Read the model definition and answer for the solid it produces. Units are mm, in the model's axes. Face numbers are marked on the shaded views. A direction names the side the tool comes from. Coordinates: 2 decimals unless noted, no trailing zeros. Order: outer loops, then holes, each group sorted by start corner. A loop starts at its lowest first (then second) coordinate and runs counter-clockwise, first axis right, second up. Notation, with made-up numbers: (39.25, 53) -> (68.25, 53) arc R22 ccw to (68.25, 64) -> close; hole circle Ø2 at (68.25, 15.25). An arc over 180 degrees is marked (long way). Use CSV: the item, a comma, the result in double quotes.
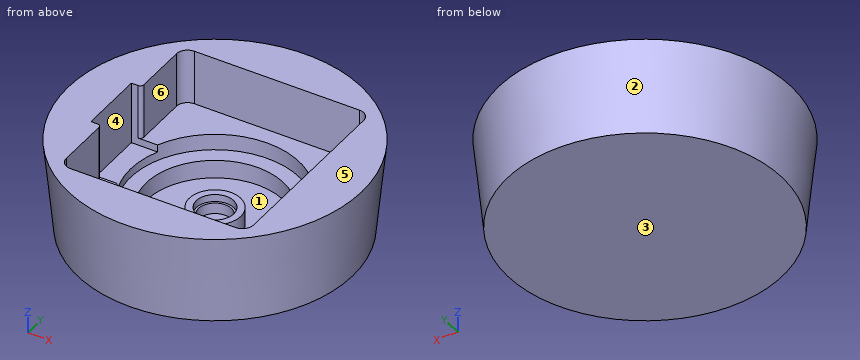
```python
from build123d import *

# Parameters (mm, degrees)
SKETCH4_W           = 51
SKETCH4_H           = 55
CUT_EXTRUDE1_DEPTH  = 15
FILLET1_R           = 3
SKETCH7_W           = 10
SKETCH7_H           = 18
CUT_EXTRUDE5_DEPTH  = 17
SKETCH8_R           = 23
CUT_EXTRUDE6_DEPTH  = 4.4
SKETCH10_R          = 18.75
CUT_EXTRUDE7_DEPTH  = 5
SKETCH11_R          = 7
BOSS_EXTRUDE3_DEPTH = 5
SKETCH12_R          = 5.1
CUT_EXTRUDE8_DEPTH  = 2
SKETCH13_R          = 4.5
CUT_EXTRUDE9_DEPTH  = 3
FILLET2_R           = 1


with BuildPart() as part:
    # Sketch2 → Revolve1 (revolve)
    with BuildSketch(Plane(origin=(0, 0, 0), x_dir=(1, 0, 0), z_dir=(0, 1, 0))):
        Polygon((0, 25), (37.5, 25), (40, 0), (0, 0), align=None)
    revolve(axis=Axis((0, 0, 0), (0, 0, -1)))

    # Sketch4 → Cut-Extrude1 (cut)
    with BuildSketch(Plane.XY):
        Rectangle(SKETCH4_W, SKETCH4_H)
    extrude(amount=-CUT_EXTRUDE1_DEPTH, mode=Mode.SUBTRACT)

    # Fillet1
    fillet1_edges = [part.edges().sort_by_distance(p)[0] for p in [
        (25.5, 27.5, -7.5),
        (25.5, -27.5, -7.5),
        (-25.5, -27.5, -7.5),
        (-25.5, 27.5, -7.5),
    ]]
    fillet(fillet1_edges, radius=FILLET1_R)

    # Sketch7 → Cut-Extrude5 (cut)
    with BuildSketch(Plane.XY):
        with Locations((-23.3, 0)):
            Rectangle(SKETCH7_W, SKETCH7_H)
    extrude(amount=-CUT_EXTRUDE5_DEPTH, mode=Mode.SUBTRACT)

    # Sketch8 → Cut-Extrude6 (cut)
    with BuildSketch(Plane.XY.offset(-15)):
        Circle(SKETCH8_R)
    extrude(amount=-CUT_EXTRUDE6_DEPTH, mode=Mode.SUBTRACT)

    # Sketch10 → Cut-Extrude7 (cut)
    with BuildSketch(Plane.XY.offset(-19.4)):
        Circle(SKETCH10_R)
    extrude(amount=-CUT_EXTRUDE7_DEPTH, mode=Mode.SUBTRACT)

    # Sketch11 → Boss-Extrude3 (add)
    with BuildSketch(Plane.XY.offset(-24.4)):
        Circle(SKETCH11_R)
    extrude(amount=BOSS_EXTRUDE3_DEPTH)

    # Sketch12 → Cut-Extrude8 (cut)
    with BuildSketch(Plane.XY.offset(-19.4)):
        Circle(SKETCH12_R)
    extrude(amount=-CUT_EXTRUDE8_DEPTH, mode=Mode.SUBTRACT)

    # Sketch13 → Cut-Extrude9 (cut)
    with BuildSketch(Plane.XY.offset(-21.4)):
        Circle(SKETCH13_R)
    extrude(amount=-CUT_EXTRUDE9_DEPTH, mode=Mode.SUBTRACT)

    # Fillet2
    fillet2_edges = [part.edges().sort_by_distance(p)[0] for p in [
        (-25.5, 9, -7.5),
        (-25.5, -9, -7.5),
    ]]
    fillet(fillet2_edges, radius=FILLET2_R)


solid = part.part
```
Item 1: A tool of negligible diameter and unlimited length cuts with its end or side. For the marked faces 5 and 6, from which of +Z, -Z, +X, -X, +Y, -Y can it reach the whole face along a straight path? Write none if from no direction.
Return value:
face 5,"+Z, +X, -X, +Y, -Y"
face 6,"+Z"
Item 2: Find section B-B, the plane y = 0. Give the vertices of the cut face in (x, z), then the cut area to 3 significant figures.
Return value:
outline,"(-40, 0) -> (-37.5, -25) -> (37.5, -25) -> (40, 0) -> (25.5, 0) -> (25.5, -15) -> (23, -15) -> (23, -19.4) -> (18.75, -19.4) -> (18.75, -24.4) -> (7, -24.4) -> (7, -19.4) -> (5.1, -19.4) -> (5.1, -21.4) -> (4.5, -21.4) -> (4.5, -24.4) -> (-4.5, -24.4) -> (-4.5, -21.4) -> (-5.1, -21.4) -> (-5.1, -19.4) -> (-7, -19.4) -> (-7, -24.4) -> (-18.75, -24.4) -> (-18.75, -19.4) -> (-23, -19.4) -> (-23, -17) -> (-28.3, -17) -> (-28.3, 0) -> close"
area,"753 mm^2"
Item 3: Each of these flat-tipped pins is pushed along its axis until it touches: P1, Ø12, axis at x = -3, z = -6, coming from the +Y side; P2, Ø6, axis at x = -24, z = -20.5, coming from the -Y side; P3, Ø3, axis at y = 25, z = -14.5, coming from the -X side. Where does it stop, or does it pass through?
Return value:
P1,"stops at y = 39.95"
P2,"stops at y = -31.64"
P3,"stops at x = -30.57"
Item 4: Find section D-D, the plane z = -7.75. Give the vertices of the cut face in (x, y) (3 decimals).
Return value:
outline,"circle Ø78.45 at (0, 0); hole (-28.3, -9) -> (-26.5, -9) arc R1 cw to (-25.5, -10) -> (-25.5, -24.5) arc R3 ccw to (-22.5, -27.5) -> (22.5, -27.5) arc R3 ccw to (25.5, -24.5) -> (25.5, 24.5) arc R3 ccw to (22.5, 27.5) -> (-22.5, 27.5) arc R3 ccw to (-25.5, 24.5) -> (-25.5, 10) arc R1 cw to (-26.5, 9) -> (-28.3, 9) -> close"
Item 5: The mould has two halves that part along Y. Classify the marked faces 1, 2, 3 and 4: +Y half, -Y half, draft (parallel to the pull), parting line (faces both ways), or undercut.
Return value:
face 1,"undercut"
face 2,"parting line"
face 3,"draft"
face 4,"undercut"
Item 6: Find section A-A, the plane z = -2.5. Give the vertices of the cut face in (x, y), then the cut area to 3 significant figures.
Return value:
outline,"circle Ø79.5 at (0, 0); hole (-28.3, -9) -> (-26.5, -9) arc R1 cw to (-25.5, -10) -> (-25.5, -24.5) arc R3 ccw to (-22.5, -27.5) -> (22.5, -27.5) arc R3 ccw to (25.5, -24.5) -> (25.5, 24.5) arc R3 ccw to (22.5, 27.5) -> (-22.5, 27.5) arc R3 ccw to (-25.5, 24.5) -> (-25.5, 10) arc R1 cw to (-26.5, 9) -> (-28.3, 9) -> close"
area,"2,120 mm^2"
Item 7: Find section C-C, the plane x = 0. Give the vertices of the cut face in (y, z).
Return value:
outline,"(-40, 0) -> (-37.5, -25) -> (37.5, -25) -> (40, 0) -> (27.5, 0) -> (27.5, -15) -> (23, -15) -> (23, -19.4) -> (18.75, -19.4) -> (18.75, -24.4) -> (7, -24.4) -> (7, -19.4) -> (5.1, -19.4) -> (5.1, -21.4) -> (4.5, -21.4) -> (4.5, -24.4) -> (-4.5, -24.4) -> (-4.5, -21.4) -> (-5.1, -21.4) -> (-5.1, -19.4) -> (-7, -19.4) -> (-7, -24.4) -> (-18.75, -24.4) -> (-18.75, -19.4) -> (-23, -19.4) -> (-23, -15) -> (-27.5, -15) -> (-27.5, 0) -> close"
Item 8: Straight lines are drawn through the part: line 1 along Y through (x, z) = (0, -20.5); line 2 along Y through (x, z) = (0, -21.9); line 3 along Z through (x, y) = (14, 1). For each, find the intervals that lie inside material, in ascending order.
Return value:
line 1,"y = -37.95 to -18.75, -7 to -5.1, 5.1 to 7, 18.75 to 37.95"
line 2,"y = -37.81 to -18.75, -7 to -4.5, 4.5 to 7, 18.75 to 37.81"
line 3,"z = -25 to -24.4"
